Can you work these out from the model? Positions are in its coordinate system, mm. Face numbers are marked on the shaded views. Give positions to 0.01 mm unless a question says otherwise; leave off trailing zeros. Order: outer loops, then holes, each group sorted by start corner. A loop starts at its lowest first (then second) coordinate and runs counter-clockwise, first axis right, second up. Notation, with made-up numbers: (27, 62) - (63, 62) arc R24 ccw to (63, 99) - close; hole circle Ø2 at (49, 85). An arc over 180 degrees is marked (long way). Answer as a JSON object with one key per item and string values.
```python
from build123d import *

# Parameters (mm, degrees)
SKETCH1_W          = 4.5
SKETCH1_H          = 28.11709914
CUT_EXTRUDE1_DEPTH = 7
CUT_EXTRUDE2_DEPTH = 7
CHAMFER1_SIZE      = 0.5
CUT_EXTRUDE3_DEPTH = 1


with BuildPart() as part:
    # Sketch1 → Revolve-Thin1 (revolve)
    with BuildSketch(Plane(origin=(0, 0, 0), x_dir=(1, 0, 0), z_dir=(0, 1, 0))):
        with Locations((2.25, 31.55854957)):
            Rectangle(SKETCH1_W, SKETCH1_H)
    revolve(axis=Axis((0, 0, 0), (0, 0, -1)))

    # Sketch2 → Cut-Extrude1 (cut)
    with BuildSketch(Plane.XY.offset(-17.5)):
        Polygon((1.610807251, 2.79), (-1.610807251, 2.79), (-3.221614502, 0), (-1.610807251, -2.79), (1.610807251, -2.79), (3.221614502, 0), align=None)
    extrude(amount=-CUT_EXTRUDE1_DEPTH, mode=Mode.SUBTRACT)

    # Sketch3 → Cut-Extrude2 (cut)
    with BuildSketch(Plane(origin=(0, 0, -45.61709914), x_dir=(-1, 0, 0), z_dir=(0, 0, -1))):
        Polygon((1.610807251, 2.79), (-1.610807251, 2.79), (-3.221614502, 0), (-1.610807251, -2.79), (1.610807251, -2.79), (3.221614502, 0), align=None)
    extrude(amount=-CUT_EXTRUDE2_DEPTH, mode=Mode.SUBTRACT)

    # Chamfer1
    chamfer1_edges = [part.edges().sort_by_distance(p)[0] for p in [
        (2.416210877, 1.395, -17.5),
        (0, 2.79, -17.5),
        (-2.416210877, 1.395, -17.5),
        (-2.416210877, -1.395, -17.5),
        (0, -2.79, -17.5),
        (2.416210877, -1.395, -17.5),
        (-2.416210877, 1.395, -45.61709914),
        (0, 2.79, -45.61709914),
        (2.416210877, 1.395, -45.61709914),
        (2.416210877, -1.395, -45.61709914),
        (0, -2.79, -45.61709914),
        (-2.416210877, -1.395, -45.61709914),
    ]]
    chamfer(chamfer1_edges, length=CHAMFER1_SIZE)

    # Sketch4 → Cut-Extrude3 (cut)
    with BuildSketch(Plane(origin=(3.897114317, 2.25, 0), x_dir=(0, 0, -1), z_dir=(0.866025404, 0.5, 0))):
        Polygon((34.73354957, 0.409595353), (34.73354957, -0.166636619), (32.087716237, 0.204797676), (32.087716237, -0.773397436), (31.55854957, -0.704707532), (31.55854957, 0.854807692), align=None)
    extrude(amount=-CUT_EXTRUDE3_DEPTH, mode=Mode.SUBTRACT)


solid = part.part
```
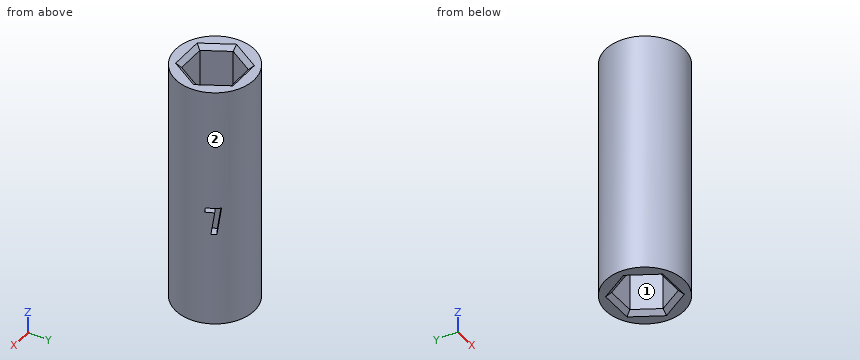
Q1. I'm going to push flat-ended pins straight in: pin 1 Ø3 at (x, z) = (-2, -37) entering from +Y; pin 2 Ø1 at (x, y) = (-1, -2.5) entering from +Z; pin 3 Ø4 at (x, y) = (-0.5, -0.5) entering from +Z. Where does each tip first touch, or does it pass through?
Recorded:
{"pin 1": "stops at y = 4.47", "pin 2": "stops at z = -17.79", "pin 3": "stops at z = -24.5"}
Q2. If we section it at B-B, the plane x = 0: Please give me the cut outline in (y, z).
Recorded:
{"outline": "(-4.5, -45.62) - (-3.29, -45.62) - (-2.79, -45.12) - (-2.79, -38.62) - (2.79, -38.62) - (2.79, -45.12) - (3.29, -45.62) - (4.5, -45.62) - (4.5, -17.5) - (3.29, -17.5) - (2.79, -18) - (2.79, -24.5) - (-2.79, -24.5) - (-2.79, -18) - (-3.29, -17.5) - (-4.5, -17.5) - close"}
Q3. I need wall thicknesses on L1, parallel to Z at x = 0.5, y = -1.75; L2, parallel to Y at x = 1.75, z = -22.25; L3, parallel to Y at x = 1.5, z = -44.5. Which ranges of each line are inside material? Lowest first, please.
Recorded:
{"L1": "z = -38.62 to -24.5", "L2": "y = -4.15 to -2.55, 2.55 to 4.15", "L3": "y = -4.24 to -2.79, 2.79 to 4.24"}
Q4. We'd pull the mould along X, two halves only. Please class the marked faces 1 and 2: released by +X, released by -X, zero draft, split by the parting line, or undercut.
Recorded:
{"face 1": "undercut", "face 2": "split by the parting line"}
Q5. If we section it at A-A, the plane z = -43: Please give me the cut outline in (x, y), then the cut area to 3 significant figures.
Recorded:
{"outline": "circle Ø9 at (0, 0); hole (-3.22, 0) - (-1.61, -2.79) - (1.61, -2.79) - (3.22, 0) - (1.61, 2.79) - (-1.61, 2.79) - close", "area": "36.7 mm^2"}
Q6. If we section it at C-C, the plane z = -26: Please give me the cut outline in (x, y).
Recorded:
{"outline": "circle Ø9 at (0, 0)"}
